Part model, mm, in its own coordinate system. Face numbers are marked on the shaded views. A direction names the side the tool comes from. Give positions to 0.01 mm unless a question says otherwise; leave off trailing zeros. Write each loop counter-clockwise with the first axis right and the second up, starting at its lowest first coordinate (ties: lowest second). Pieces come first, ordered by that corner, then holes. Notation, with made-up numbers: (13.25, 3) - (32.25, 3) arc R26 cw to (32.25, 33) - close; hole circle Ø8 at (68, 41.25). An arc over 180 degrees is marked (long way). Answer as a JSON object with one key per item and string values. Group by question number.
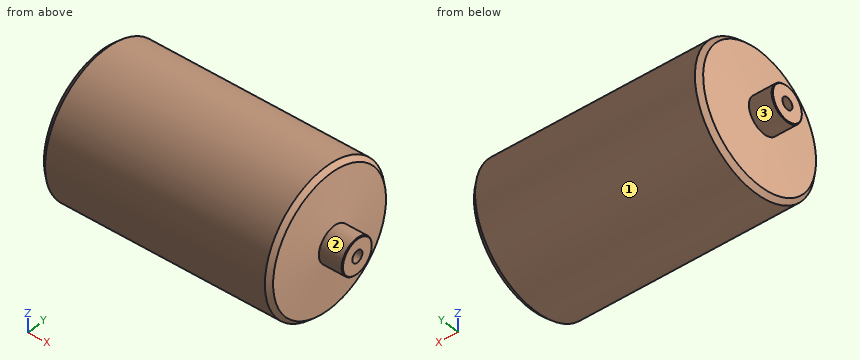
```python
from build123d import *

# Parameters (mm, degrees)
CHAMFER_1_SIZE      = 3
CHAMFER_2_SIZE      = 0.5
HOLE_WIZARD_1_D     = 8.376
HOLE_WIZARD_1_DEPTH = 59
HOLE_WIZARD_1_TIP   = 2.516404272
HOLE_WIZARD_2_D     = 8.376
HOLE_WIZARD_2_DEPTH = 59
HOLE_WIZARD_2_TIP   = 2.516404272


with BuildPart() as part:
    # 草圖1 → 迴轉1 (revolve)
    with BuildSketch(Plane.XY, mode=Mode.PRIVATE) as revolve_1_sk:
        Polygon((0, 0), (0, 12.5), (16.5, 12.5), (19.780824882, 50), (180.219175118, 50), (183.5, 12.5), (200, 12.5), (200, 0), align=None)
    revolve(revolve_1_sk.sketch.rotate(Axis((0, 0, 0), (1, 0, 0)), 90), axis=Axis((0, 0, 0), (1, 0, 0)))

    # 倒角1
    chamfer_1_edges = [part.edges().sort_by_distance(p)[0] for p in [
        (180.219175118, 0, -50),
        (19.780824882, 0, -50),
    ]]
    chamfer(chamfer_1_edges, length=CHAMFER_1_SIZE)

    # 倒角2
    chamfer_2_edges = [part.edges().sort_by_distance(p)[0] for p in [
        (200, 0, -12.5),
        (0, 0, -12.5),
    ]]
    chamfer(chamfer_2_edges, length=CHAMFER_2_SIZE)

    # 孔1
    with Locations(Plane(origin=(200, 0, 0), x_dir=(0, 0, -1), z_dir=(1, 0, 0))):
        with Locations((0, 0)):
            Hole(HOLE_WIZARD_1_D / 2, depth=HOLE_WIZARD_1_DEPTH)
            with Locations((0, 0, -(HOLE_WIZARD_1_DEPTH + HOLE_WIZARD_1_TIP / 2))):  # 118° drill point
                Cone(0, HOLE_WIZARD_1_D / 2, HOLE_WIZARD_1_TIP, mode=Mode.SUBTRACT)

    # 孔2
    with Locations(Plane.ZY):
        with Locations((0, 0)):
            Hole(HOLE_WIZARD_2_D / 2, depth=HOLE_WIZARD_2_DEPTH)
            with Locations((0, 0, -(HOLE_WIZARD_2_DEPTH + HOLE_WIZARD_2_TIP / 2))):  # 118° drill point
                Cone(0, HOLE_WIZARD_2_D / 2, HOLE_WIZARD_2_TIP, mode=Mode.SUBTRACT)


solid = part.part
```
1) Drop flat-ended pins along their axis: P1, Ø8, axis at x = 169.5, z = 7.5, coming from the +Y side; P2, Ø1, axis at x = 149, z = -23, coming from the -Y side; P3, Ø2, axis at x = 52, y = -15.5, coming from the -Z side. Give the stop position or say it passes through.
2) Which spindle directions (+Z, -Z, +X, -X, +Y, -Y) get a long thin tool onto all of the face, cutting with end or side? Do the marked faces 1, 2 and 3. Say none if no direction does.
3) Drill centre lines: line 1 along Y through (x, z) = (36, 0); line 2 along Y through (x, z) = (34.5, -3); line 3 along Z through (x, y) = (109.5, -30.5). Where is each one in solid material? Low to high. Write a range as from..to.
4) Saw through at A-A (x = 134.5). List the corners of the cut face in (y, z).
Checks:
{
 "1": {"P1": "y = 49.88", "P2": "y = -44.65", "P3": "z = -47.85"},
 "2": {"face 1": "+X, -X", "face 2": "+X", "face 3": "-X"},
 "3": {"line 1": "-50..-4.19, 4.19..50", "line 2": "-49.91..-2.92, 2.92..49.91", "line 3": "-39.62..39.62"},
 "4": {"outline": "circle Ø100 at (0, 0)"}
}
